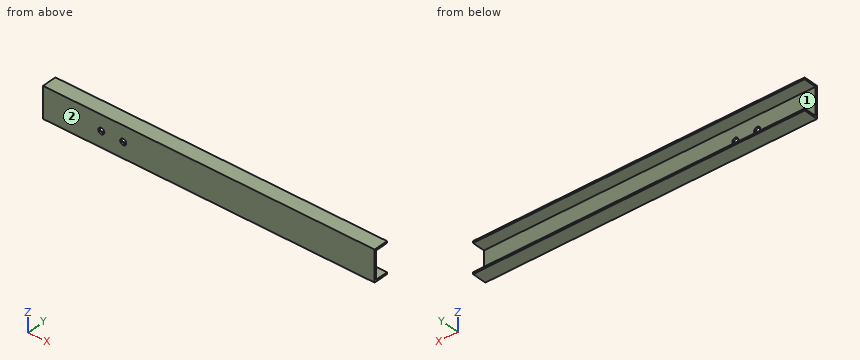
```python
from build123d import *

# Parameters (mm, degrees)
SKETCH1_W               = 182
SKETCH1_H               = 17
BOSS_EXTRUDE1_DEPTH     = 1
SKETCH8_W               = 182
SKETCH8_H               = 1
BOSS_EXTRUDE2_DEPTH     = 7
ADVANCEDHOLE1_OUTLINE_R = 1.65
ADVANCEDHOLE1_DEPTH     = 1
SKETCH12_W              = 182
SKETCH12_H              = 13
SKETCH12_R              = 2
BOSS_EXTRUDE3_DEPTH     = 1
SKETCH13_W              = 182
SKETCH13_H              = 1
BOSS_EXTRUDE4_DEPTH     = 3


# Read off the part's stored shape, not the designer's step: AdvancedHole1
with BuildPart() as part:
    # Sketch1 → Boss-Extrude1 (new body)
    with BuildSketch(Plane(origin=(0, 0, 0), x_dir=(1, 0, 0), z_dir=(0, 1, 0))):
        Rectangle(SKETCH1_W, SKETCH1_H)
    extrude(amount=BOSS_EXTRUDE1_DEPTH)

    # Sketch8 → Boss-Extrude2 (add)
    with BuildSketch(Plane(origin=(0, 1, 0), x_dir=(1, 0, 0), z_dir=(0, 1, 0))):
        with Locations((0, 8)):
            Rectangle(SKETCH8_W, SKETCH8_H)
        with Locations((0, -8)):
            Rectangle(SKETCH8_W, SKETCH8_H)
    extrude(amount=BOSS_EXTRUDE2_DEPTH)

    # AdvancedHole1 outline → AdvancedHole1 (cut)
    with BuildSketch(Plane(origin=(0, 0, 0), x_dir=(1, 0, 0), z_dir=(0, 1, 0))):
        with Locations((-47, 0)):
            Circle(ADVANCEDHOLE1_OUTLINE_R)
        with Locations((-59, 0)):
            Circle(ADVANCEDHOLE1_OUTLINE_R)
    extrude(amount=ADVANCEDHOLE1_DEPTH, mode=Mode.SUBTRACT)


with BuildPart() as body_2:
    # Sketch12 → Boss-Extrude3 (new body)
    with BuildSketch(Plane(origin=(0, 0, 0), x_dir=(1, 0, 0), z_dir=(0, 1, 0))):
        with Locations((0, 44.153691451)):
            Rectangle(SKETCH12_W, SKETCH12_H)
        with Locations(Location((-72, 44.153691451, 0), (0, 0, 270))):
            Circle(SKETCH12_R, mode=Mode.SUBTRACT)
        with Locations(Location((-64, 44.153691451, 0), (0, 0, 270))):
            Circle(SKETCH12_R, mode=Mode.SUBTRACT)
        with Locations(Location((-56, 44.153691451, 0), (0, 0, 270))):
            Circle(SKETCH12_R, mode=Mode.SUBTRACT)
        with Locations(Location((-40, 44.153691451, 0), (0, 0, 270))):
            Circle(SKETCH12_R, mode=Mode.SUBTRACT)
        with Locations(Location((-32, 44.153691451, 0), (0, 0, 270))):
            Circle(SKETCH12_R, mode=Mode.SUBTRACT)
        with Locations(Location((-24, 44.153691451, 0), (0, 0, 270))):
            Circle(SKETCH12_R, mode=Mode.SUBTRACT)
        with Locations(Location((40, 44.153691451, 0), (0, 0, 90))):
            Circle(SKETCH12_R, mode=Mode.SUBTRACT)
        with Locations(Location((32, 44.153691451, 0), (0, 0, 90))):
            Circle(SKETCH12_R, mode=Mode.SUBTRACT)
        with Locations(Location((24, 44.153691451, 0), (0, 0, 90))):
            Circle(SKETCH12_R, mode=Mode.SUBTRACT)
        with Locations(Location((8, 44.153691451, 0), (0, 0, 90))):
            Circle(SKETCH12_R, mode=Mode.SUBTRACT)
        with Locations(Location((0, 44.153691451, 0), (0, 0, 90))):
            Circle(SKETCH12_R, mode=Mode.SUBTRACT)
        with Locations(Location((-8, 44.153691451, 0), (0, 0, 90))):
            Circle(SKETCH12_R, mode=Mode.SUBTRACT)
        with Locations(Location((72, 44.153691451, 0), (0, 0, 270))):
            Circle(SKETCH12_R, mode=Mode.SUBTRACT)
        with Locations(Location((64, 44.153691451, 0), (0, 0, 270))):
            Circle(SKETCH12_R, mode=Mode.SUBTRACT)
        with Locations(Location((56, 44.153691451, 0), (0, 0, 270))):
            Circle(SKETCH12_R, mode=Mode.SUBTRACT)
    extrude(amount=BOSS_EXTRUDE3_DEPTH)

    # Sketch13 → Boss-Extrude4 (add)
    with BuildSketch(Plane(origin=(0, 1, 0), x_dir=(1, 0, 0), z_dir=(0, 1, 0))):
        with Locations((0, 50.153691451)):
            Rectangle(SKETCH13_W, SKETCH13_H)
        with Locations((0, 38.153691451)):
            Rectangle(SKETCH13_W, SKETCH13_H)
    extrude(amount=BOSS_EXTRUDE4_DEPTH)


solid = part.part
```
Verification items for the finished model (mm, model axes). Face numbers are marked on the shaded views. Round coordinates to 2 decimals unless told otherwise and drop trailing zeros. Write each loop counter-clockwise with the first axis right and the second up, starting at its lowest first coordinate (ties: lowest second). Pieces come first, ordered by that corner, then holes. Notation, with made-up numbers: (-28.75, 87.25) - (0.25, 87.25) arc R17 ccw to (0.25, 105.25) - close; hole circle Ø6 at (-13, 46). An arc over 180 degrees is marked (long way). Answer as a JSON object with one key per item and string values. Group by question number.
Q1. Section check B-B, the plane x = -47. Enter the section's corners in (y, z).
Q2. Section check A-A, the plane z = 0. Enter the section's corners in (x, y), plus the area to 3 significant figures.
Q3. Thickness scan on line 1 (X direction, y = 0.25, z = 0); line 2 (Z direction, x = 22, y = 6.5); line 3 (Z direction, x = -59, y = 0.4). Record the ranges inside material, lowest first.
Q4. Section check C-C, the plane y = 2.25. Enter the section's corners in (x, z).
Q5. Section check D-D, the plane x = 31. Enter the section's corners in (y, z), plus the area to 3 significant figures.
Q6. Mould release check, pull along Z, two halves, no side actions. Record for the marked faces 1 and 2: released by +Z, released by -Z, zero draft, split by the parting line, or undercut.
Found:
{
 "1": {"outline": "(0, -8.5) - (8, -8.5) - (8, -7.5) - (1, -7.5) - (1, -1.65) - (0, -1.65) - close; (0, 1.65) - (1, 1.65) - (1, 7.5) - (8, 7.5) - (8, 8.5) - (0, 8.5) - close"},
 "2": {"outline": "(-91, 0) - (-60.65, 0) - (-60.65, 1) - (-91, 1) - close; (-57.35, 0) - (-48.65, 0) - (-48.65, 1) - (-57.35, 1) - close; (-45.35, 0) - (91, 0) - (91, 1) - (-45.35, 1) - close", "area": "175 mm^2"},
 "3": {"line 1": "x = -91 to -60.65, -57.35 to -48.65, -45.35 to 91", "line 2": "z = -8.5 to -7.5, 7.5 to 8.5", "line 3": "z = -8.5 to -1.65, 1.65 to 8.5"},
 "4": {"outline": "(-91, -8.5) - (91, -8.5) - (91, -7.5) - (-91, -7.5) - close; (-91, 7.5) - (91, 7.5) - (91, 8.5) - (-91, 8.5) - close"},
 "5": {"outline": "(0, -8.5) - (8, -8.5) - (8, -7.5) - (1, -7.5) - (1, 7.5) - (8, 7.5) - (8, 8.5) - (0, 8.5) - close", "area": "31.0 mm^2"},
 "6": {"face 1": "undercut", "face 2": "zero draft"}
}
